```python
from build123d import *

# Parameters (mm, degrees)
BOSS_EXTRUDE1_DEPTH      = 10
BOSS_EXTRUDE2_DEPTH      = 30
BOSS_EXTRUDE2_DEPTH_BACK = 50
SKETCH2_R                = 12.5
SKETCH3_R                = 17.5
BOSS_EXTRUDE3_DEPTH      = 20
FILLET1_R                = 3
SKETCH4_R                = 1.5
CUT_EXTRUDE1_DEPTH       = 10


with BuildPart() as part:
    # Sketch1 → Boss-Extrude1 (new body)
    with BuildSketch(Plane(origin=(0, 0, 0), x_dir=(1, 0, 0), z_dir=(0, 1, 0))):
        with BuildLine():
            Line((-50.126401, 19.839202), (-7.169705, -10.239401))
            ThreePointArc((-7.169705, -10.239401), (0, -12.5), (7.169705, -10.239401))
            Line((7.169705, -10.239401), (50.126401, 19.839202))
            ThreePointArc((50.126401, 19.839202), (54.194564, 26.060188), (52.845996, 33.369907))
            ThreePointArc((52.845996, 33.369907), (0, 62.5), (-52.845996, 33.369907))
            ThreePointArc((-52.845996, 33.369907), (-54.194564, 26.060188), (-50.126401, 19.839202))
        make_face()
    extrude(amount=BOSS_EXTRUDE1_DEPTH)

    # Sketch2 → Boss-Extrude2 (add, two sides: drawn at the far end of the back side and taken through both)
    with BuildSketch(Plane(origin=(0, 10, 0), x_dir=(1, 0, 0), z_dir=(0, 1, 0)).offset(-BOSS_EXTRUDE2_DEPTH_BACK)):
        with Locations(Location((0, 0, 0), (0, 0, 270))):
            Circle(SKETCH2_R)
    extrude(amount=BOSS_EXTRUDE2_DEPTH + BOSS_EXTRUDE2_DEPTH_BACK)

    # Sketch3 → Boss-Extrude3 (add)
    with BuildSketch(Plane.XZ):
        with Locations(Location((0, 0, 0), (0, 0, 169.415309))):
            Circle(SKETCH3_R)
    extrude(amount=BOSS_EXTRUDE3_DEPTH)

    # Fillet1
    fillet1_edges = [part.edges().sort_by_distance(p)[0] for p in [
        (0, 40, -12.5),
    ]]
    fillet(fillet1_edges, radius=FILLET1_R)

    # Sketch4 → Cut-Extrude1 (cut)
    with BuildSketch(Plane.XZ.offset(40)):
        with Locations(Location((0, 9, 0), (0, 0, 270))):
            Circle(SKETCH4_R)
        with Locations(Location((9, 0, 0), (0, 0, 270))):
            Circle(SKETCH4_R)
        with Locations(Location((0, -9, 0), (0, 0, 270))):
            Circle(SKETCH4_R)
        with Locations(Location((-9, 0, 0), (0, 0, 270))):
            Circle(SKETCH4_R)
    extrude(amount=-CUT_EXTRUDE1_DEPTH, mode=Mode.SUBTRACT)


solid = part.part
```
Source: CAD feature listing. Evaluate the final solid. Frame: model axes, mm. A direction names the side the tool comes from. Give positions to 0.01 mm unless a question says otherwise; leave off trailing zeros. Write each loop counter-clockwise with the first axis right and the second up, starting at its lowest first coordinate (ties: lowest second). Pieces come first, ordered by that corner, then holes. Notation, with made-up numbers: (-0.5, 9.5) - (27.5, 9.5) arc R15 ccw to (27.5, 19.5) - close; hole circle Ø8 at (-16.75, 21.25). An arc over 180 degrees is marked (long way). One line per item, written item: value. Start each with the question number.
Q1. Draft query along Z for faces 4 (the face through (-28.95, 4.93, -5.01)), 5 (the face through (3.755, -30.14, 11.923)), 6 (the face through (0, -30, 9)). Return one class per face: +Z half, -Z half, draft (parallel to the pull), parting line (faces both ways), or undercut.
Q2. Section query D-D, the plane y = -7.5. Return the cut outline in (x, z), then the cut area to 3 significant figures.
Q3. Section query A-A, the plane y = -32.5. Return the cut outline in (x, z), then the cut area to 3 significant figures.
Q4. Set-up query: faces 1 (the face through (9, -30, 0)), 2 (the face through (-1, 0, 13)), 3 (the face through (28.35, 4.93, -4.59)). Return all of +Z, -Z, +X, -X, +Y, -Y with unobstructed straight access to the full face (end or side cutting, diameter ignored); none if empty.
Q5. Section query C-C, the plane z = 0. Return the cut outline in (x, y), then the cut area to 3 significant figures.
Q6. Material intervals for probe 1 along X at (y, z) = (-35.5, 0); probe 2 along Y at (x, z) = (20, -48.5); probe 3 along X at (y, z) = (-36.5, -9), sorted ascending. Write a range as from..to.
Q7. First-contact query: pin 1 Ø3.5 at (x, z) = (9.5, 0.5) entering from -Y; pin 2 Ø12 at (x, z) = (8.5, -16.5) entering from +Y; pin 3 Ø2.5 at (x, z) = (0, -9) entering from -Y; pin 4 Ø3 at (y, z) = (27.5, 6) entering from -X. Flat tips, straight axial feed; report the tip coordinate or a pass-through.
Q8. Section query B-B, the plane x = 0. Return the cut outline in (y, z).
Answer:
1. face 4: +Z half
1. face 5: parting line
1. face 6: undercut
2. outline: circle Ø35 at (0, 0)
2. area: 962 mm2
3. outline: circle Ø25 at (0, 0); hole circle Ø3 at (-9, 0); hole circle Ø3 at (0, -9); hole circle Ø3 at (0, 9); hole circle Ø3 at (9, 0)
3. area: 463 mm2
4. face 1: -Y
4. face 2: +Z, +Y
4. face 3: +Z, +X, +Y
5. outline: (-21.79, 0) - (-17.5, 0) - (-17.5, -20) - (-12.5, -20) - (-12.5, -40) - (-10.5, -40) - (-10.5, -30) - (-7.5, -30) - (-7.5, -40) - (7.5, -40) - (7.5, -30) - (10.5, -30) - (10.5, -40) - (12.5, -40) - (12.5, -20) - (17.5, -20) - (17.5, 0) - (21.79, 0) - (21.79, 10) - (12.5, 10) - (12.5, 37) arc R3 ccw to (9.5, 40) - (-9.5, 40) arc R3 ccw to (-12.5, 37) - (-12.5, 10) - (-21.79, 10) - close
5. area: 2,320 mm2
6. probe 1: x = -12.5..-10.5, -7.5..7.5, 10.5..12.5
6. probe 2: y = 0..10
6. probe 3: x = -8.67..-1.5, 1.5..8.67
7. pin 1: stops at y = -40
7. pin 2: stops at y = 10
7. pin 3: stops at y = -30
7. pin 4: stops at x = -11.66
8. outline: (-40, -12.5) - (-20, -12.5) - (-20, -17.5) - (0, -17.5) - (0, -62.5) - (10, -62.5) - (10, -12.5) - (37, -12.5) arc R3 ccw to (40, -9.5) - (40, 9.5) arc R3 ccw to (37, 12.5) - (0, 12.5) - (0, 17.5) - (-20, 17.5) - (-20, 12.5) - (-40, 12.5) - (-40, 10.5) - (-30, 10.5) - (-30, 7.5) - (-40, 7.5) - (-40, -7.5) - (-30, -7.5) - (-30, -10.5) - (-40, -10.5) - close
